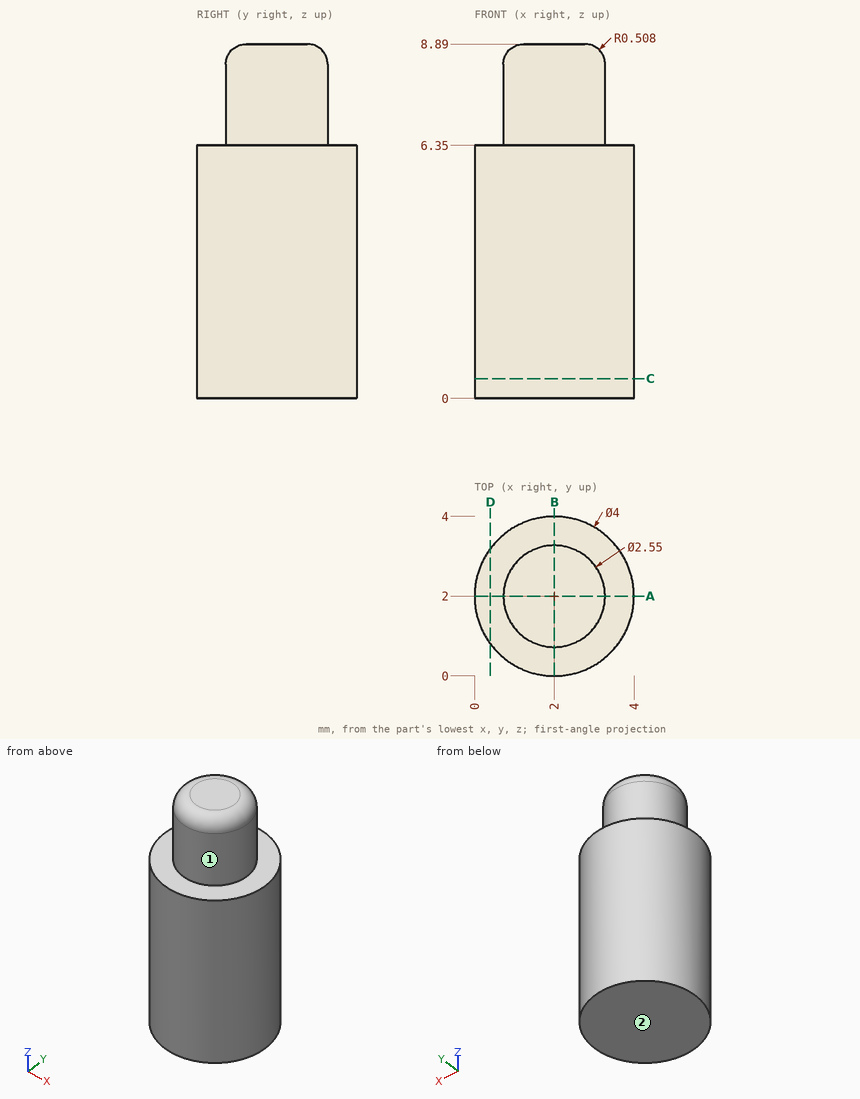
For this review, use the dimensioned drawing (mm, ordinates from the lowest corner) and the shaded views. A direction names the side the tool comes from. Coordinates: 2 decimals unless noted, no trailing zeros. Loops run counter-clockwise (first coordinate to the right, second up) from the corner with the lowest first, then second, coordinate; pieces in that order, holes last. Notation, with made-up numbers: (43.25, 83) -> (73.25, 83) arc R6 ccw to (73.25, 92) -> close; hole circle Ø5 at (-17.5, 80). An arc over 180 degrees is marked (long way). Use a Markdown table: item, result. Add a question column.
1. To check wall thickness, follow line 1 (Z direction, x = 1.15, y = 3.75); line 2 (Y direction, x = 1.9, z = 3); line 3 (X direction, y = 2.15, z = 0.5). State the ranges of each line that lie inside material, in increasing order.
2. Add section A-A on y = 2. Write out the cut boundary in (x, z) (3 decimals).
3. Machinability: for the marked faces 1 and 2, which of the approach directions +Z, -Z, +X, -X, +Y, -Y give a long, thin tool a straight path to every point of the face, cutting with its end or side? Answer none if there is none.
4. Add section C-C on z = 0.5. Write out the cut boundary in (x, y), plus the area to 3 significant figures.
5. Add section D-D on x = 0.4. Write out the cut boundary in (y, z), plus the area to 3 significant figures.
Returned:
| question | item | result |
|---|---|---|
| 1 | line 1 | z = 0 to 6.35 |
| 1 | line 2 | y = 0 to 4 |
| 1 | line 3 | x = 0.01 to 3.99 |
| 2 | outline | (0, 0) -> (4, 0) -> (4, 6.35) -> (3.275, 6.35) -> (3.275, 8.382) arc R0.508 ccw to (2.767, 8.89) -> (1.233, 8.89) arc R0.508 ccw to (0.725, 8.382) -> (0.725, 6.35) -> (0, 6.35) -> close |
| 3 | face 1 | +Z |
| 3 | face 2 | -Z, +X, -X, +Y, -Y |
| 4 | outline | circle Ø4 at (2, 2) |
| 4 | area | 12.6 mm² |
| 5 | outline | (0.8, 0) -> (3.2, 0) -> (3.2, 6.35) -> (0.8, 6.35) -> close |
| 5 | area | 15.2 mm² |
